Check sheet for the modelled part. Datum: model origin and axes. Units: mm. Face numbers are marked on the shaded views. A direction names the side the tool comes from. Coordinates: 2 decimals unless noted, no trailing zeros. Loops run counter-clockwise (first coordinate to the right, second up) from the corner with the lowest first, then second, coordinate; pieces in that order, holes last. Notation, with made-up numbers: (-27, 69) -> (9, 69) arc R22 cw to (9, 84) -> close; hole circle Ø5 at (40, 12). An arc over 180 degrees is marked (long way). Use one line per item in the form item = value.
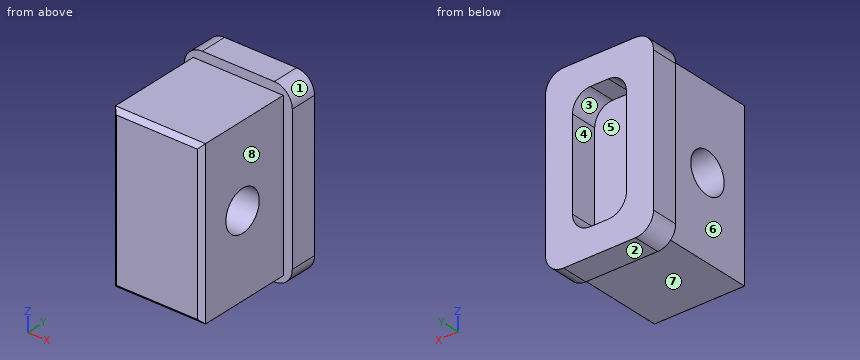
Autodesk Inventor part; units mm, degrees
ref_plane "YZ Plane" through (0, 0, 0) normal (1, 0, 0) x (0, 1, 0)
ref_plane "XZ Plane" through (0, 0, 0) normal (0, 1, 0) x (-1, 0, 0)
ref_plane "XY Plane" through (0, 0, 0) normal (0, 0, 1) x (1, 0, 0)
sketch "Sketch1" plane through (0, 0, 0) normal (0, 1, 0) x (-1, 0, 0)
  line L0 (0, 0) -> (-12, 0)
  line L1 (-12, 0) -> (-12, -20)
  line L2 (-12, -20) -> (0, -20)
  line L3 (0, -20) -> (0, 0)
  line L4 (-6, 0) -> (-6, -1)
  line L5 (-6, -1) -> (-1, -1)
  line L6 (-1, -1) -> (-11, -1)
  line L7 (-11, -1) -> (-11, -19)
  line L8 (-11, -19) -> (-1, -19)
  line L9 (-1, -19) -> (-1, -1)
  dimension "d0" = 12
  dimension "d1" = 20
  dimension "d2" = 1
  dimension "d3" = 5
  dimension "d4" = 10
  dimension "d5" = 18
  dimension "d35" = 0
  dimension "d36" = 1
extrude "Extrusion1" add sketch "Sketch1" along normal blind 3
sketch "Sketch2" plane through (0, 3, 0) normal (0, 1, 0) x (1, 0, 0)
  line L0 (11, 1) -> (1, 1)
  line L1 (11, 19) -> (11, 1)
  line L2 (1, 1) -> (11, 1)
  line L3 (11, 1) -> (11, 19)
  line L4 (11, 19) -> (1, 19)
  line L5 (1, 19) -> (1, 1)
  point P0 (0, 0)
  point P1 (0, 0)
  dimension "d37" = 10
  dimension "d38" = 18
  dimension "d39" = 11
  dimension "d40" = 19
  dimension "d41" = 11
  dimension "d42" = 1
extrude "Extrusion4" add sketch "Sketch2" against normal blind 14
sketch "Sketch5" plane through (11, -11, -1) normal (1, 0, 0) x (0, 0, -1)
  line L0 (0, 11) -> (18, 11)
  line L1 (0, 11) -> (0, 0)
  line L2 (18, 0) -> (0, 0)
  line L3 (18, 11) -> (18, 0)
  circle A0 centre (9, 5.5) radius 2.25
  point P0 (-1, 11)
  dimension "d21" = 4.5
  dimension "d43" = 9
  dimension "d44" = 5.5
extrude "Extrusion5" cut sketch "Sketch5" against normal through all contours A0
sketch "Sketch6" plane through (0, 3, 0) normal (0, 1, 0) x (1, 0, 0)
  line L0 (6, 0) -> (6, 3)
  line L1 (6, 3) -> (6, 17)
  line L2 (6, 3) -> (3, 3)
  line L3 (3, 3) -> (3, 17)
  line L4 (3, 17) -> (9, 17)
  line L5 (9, 17) -> (9, 3)
  line L6 (9, 3) -> (6, 3)
  point P0 (0, 0)
  point P1 (0, 0)
  dimension "d24" = 3
  dimension "d25" = 14
  dimension "d26" = 3
  dimension "d27" = 6
  dimension "d28" = 14
  dimension "d29" = 9
  dimension "d30" = 3
  dimension "d31" = 9
  dimension "d32" = 3
extrude "Extrusion6" cut sketch "Sketch6" against normal blind 3
chamfer "Chamfer1" distance 0.5 angle 45 4 edges at (11, -11, -10) (1, -11, -10) (6, -11, -1) (6, -11, -19)
fillet "Fillet1" radius 2 4 edges at (12, 1.5, -20) (12, 1.5, 0) (0, 1.5, -20) (0, 1.5, 0)
fillet "Fillet2" radius 2 4 edges at (3, 1.5, -3) (3, 1.5, -17) (9, 1.5, -3) (9, 1.5, -17)
properties part number "reverse gear steam chest side valve"
(1) Tool access check on the marked faces 5, 6, 7 and 8. Record the directions out of +Z, -Z, +X, -X, +Y, -Y that give a thin tool (end or side, any length) a straight path to the whole face; none if there is none.
Established:
face_5 = +Y
face_6 = +Z, -Z, -X, -Y
face_7 = -Z, +X, -X, -Y
face_8 = +Z, -Z, +X, -Y
(2) Section check D-D, the plane z = -13. Record the boundary of the cut face in (x, y), plus the area to 3 significant figures.
Established:
outline = (0, 0) -> (1, 0) -> (1, -10.5) -> (1.5, -11) -> (10.5, -11) -> (11, -10.5) -> (11, 0) -> (12, 0) -> (12, 3) -> (9, 3) -> (9, 0) -> (3, 0) -> (3, 3) -> (0, 3) -> close
area = 128 mm²
(3) Section check C-C, the plane y = 1.5. Record the boundary of the cut face in (x, z).
Established:
outline = (0, -18) arc R2 ccw to (2, -20) -> (10, -20) arc R2 ccw to (12, -18) -> (12, -2) arc R2 ccw to (10, 0) -> (2, 0) arc R2 ccw to (0, -2) -> close; hole (3, -15) arc R2 ccw to (5, -17) -> (7, -17) arc R2 ccw to (9, -15) -> (9, -5) arc R2 ccw to (7, -3) -> (5, -3) arc R2 ccw to (3, -5) -> close
(4) Scan lines: line 1 along X through (y, z) = (1.75, -11.5); line 2 along X through (y, z) = (-3.75, -16); line 3 along Z through (x, y) = (3.25, -7.5). Record each from-to range of solid material in increasing order.
Established:
line_1 = 0 to 3, 9 to 12
line_2 = 1 to 11
line_3 = -19 to -11.03, -8.97 to -1
(5) Section check A-A, the plane y = -5.5. Record the boundary of the cut face in (x, z).
Established:
outline = (1, -19) -> (11, -19) -> (11, -12.25) -> (1, -12.25) -> close; (1, -7.75) -> (11, -7.75) -> (11, -1) -> (1, -1) -> close
(6) Mould release check, pull along Z, two halves, no side actions. Record for the marked faces 1, 2, 3 and 4: +Z half, -Z half, draft (parallel to the pull), parting line (faces both ways), or undercut.
Established:
face_1 = +Z half
face_2 = -Z half
face_3 = undercut
face_4 = undercut
(7) Section check B-B, the plane z = -10. Record the boundary of the cut face in (x, y).
Established:
outline = (0, 0) -> (1, 0) -> (1, -3.25) -> (11, -3.25) -> (11, 0) -> (12, 0) -> (12, 3) -> (9, 3) -> (9, 0) -> (3, 0) -> (3, 3) -> (0, 3) -> close; (1, -10.5) -> (1.5, -11) -> (10.5, -11) -> (11, -10.5) -> (11, -7.75) -> (1, -7.75) -> close
(8) Go/stop test with flat-tipped pins: P1, Ø4, axis at x = 5, y = -7.5, coming from the -Z side; P2, Ø3, axis at y = -4, z = -12.5, coming from the +X side; P3, Ø1, axis at x = 6.5, z = -4.5, coming from the +Y side; P4, Ø2.5, axis at y = -5.5, z = -10, coming from the +X side. Record where each tip stops, or that it passes through.
Established:
P1 = -19
P2 = 11
P3 = 0
P4 = through
